from build123d import *

# Parameters (mm, degrees)
BOSS_EXTRU_1_DEPTH   = 6
EMPREINTE1_OUTLINE_W = 6
EMPREINTE1_OUTLINE_H = 18
EMPREINTE1_DEPTH     = 6


# Read off the part's stored shape, not the designer's step: Empreinte1
with BuildPart() as part:
    # Esquisse1 → Boss.-Extru.1 (new body)
    with BuildSketch(Plane.XY):
        Polygon((-286.806510123, 2.22734392), (-90.921937441, 115.321354688), (51.5, 33.094010768), (51.5, -193.094010768), (-90.921937441, -275.321354688), (-286.806510123, -162.22734392), align=None)
        Polygon((-246.806510123, -139.133333153), (-246.806510123, -20.866666847), (-90.921937441, 69.133333153), (11.5, 10), (11.5, -170), (-90.921937441, -229.133333153), align=None, mode=Mode.SUBTRACT)
    extrude(amount=BOSS_EXTRU_1_DEPTH)

    # Empreinte1 outline → Empreinte1 (cut)
    with BuildSketch(Plane.XY):
        Polygon((-6.833974392, -200.800909817), (-3.833974392, -205.99706224), (11.754482876, -196.99706224), (8.754482876, -191.800909817), align=None)
        Polygon((-22.42243166, -209.800909817), (-38.010888928, -218.800909817), (-35.010888928, -223.99706224), (-19.42243166, -214.99706224), align=None)
        Polygon((-53.599346196, -227.800909817), (-69.187803464, -236.800909817), (-66.187803464, -241.99706224), (-50.599346196, -232.99706224), align=None)
        with Locations((-266.319584862, -116.867002045)):
            Rectangle(EMPREINTE1_OUTLINE_W, EMPREINTE1_OUTLINE_H)
        with Locations((-266.319584862, -80.867002045)):
            Rectangle(EMPREINTE1_OUTLINE_W, EMPREINTE1_OUTLINE_H)
        with Locations((-266.319584862, -44.867002045)):
            Rectangle(EMPREINTE1_OUTLINE_W, EMPREINTE1_OUTLINE_H)
        Polygon((-54.593654623, 67.789098441), (-51.593654623, 72.985250863), (-67.182111891, 81.985250863), (-70.182111891, 76.789098441), align=None)
        Polygon((-39.005197355, 58.789098441), (-23.416740087, 49.789098441), (-20.416740087, 54.985250863), (-36.005197355, 63.985250863), align=None)
        Polygon((-7.828282819, 40.789098441), (7.76017445, 31.789098441), (10.76017445, 36.985250863), (-4.828282819, 45.985250863), align=None)
    extrude(amount=EMPREINTE1_DEPTH, mode=Mode.SUBTRACT)


solid = part.part
Verification items for the finished model (mm, model axes). A direction names the side the tool comes from. Coordinates: 2 decimals unless noted, no trailing zeros. Order: outer loops, then holes, each group sorted by start corner. A loop starts at its lowest first (then second) coordinate and runs counter-clockwise, first axis right, second up.
Item 1: Section check D-D, the plane z = 5. Give the number of separate pieces and of enclosed holes in the cut face, then the cut area to 3 significant figures.
Filled in:
separate pieces: 1
enclosed holes: 10
area: 40,400 mm2
Item 2: Release check for a two-part mould opening along X. For faces 1 (the face through (-154, -195, 6)), 2 (the face through (-190.24, 57.98, 2.96)), 3 (the face through (-59.279, 77.422, 2.958)) record: +X half, -X half, draft (parallel to the pull), parting line (faces both ways), or undercut.
Filled in:
face 1: draft
face 2: -X half
face 3: undercut
Item 3: Section check B-B, the plane x = -212.5. Enter the section's corners in (y, z).
Filled in:
outline: (-205.13, 0) - (-158.94, 0) - (-158.94, 6) - (-205.13, 6) - close; (-1.06, 0) - (45.13, 0) - (45.13, 6) - (-1.06, 6) - close
Item 4: Section check C-C, the plane y = -4. Enter the section's corners in (x, z), then the cut area to 3 significant figures.
Filled in:
outline: (-286.81, 0) - (-217.59, 0) - (-217.59, 6) - (-286.81, 6) - close; (11.5, 0) - (51.5, 0) - (51.5, 6) - (11.5, 6) - close
area: 655 mm2
Item 5: Access from +Z, -Z, +X, -X, +Y, -Y to the whole of each face (thin tool, end or side, straight path). Record for faces 4 (the face through (-18.71, -233.63, 2.96)), 5 (the face through (-0.14, 36.35, 2.96)).
Filled in:
face 4: +Z, -Z, +X, -Y
face 5: +Z, -Z
Item 6: Section check A-A, the plane y = -43.5. Enter the section's corners in (x, z).
Filled in:
outline: (-286.81, 0) - (-269.32, 0) - (-269.32, 6) - (-286.81, 6) - close; (-263.32, 0) - (-246.81, 0) - (-246.81, 6) - (-263.32, 6) - close; (11.5, 0) - (51.5, 0) - (51.5, 6) - (11.5, 6) - close
Item 7: Depth check by flat-ended pin: pin 1 (1.8 mm diameter, centred on x = -265.5, z = 3, fed in from -Y); pin 2 (3 mm diameter, centred on x = -266.5, z = 2.5, fed in from -Y); pin 3 (3 mm diameter, centred on x = -266, z = 4, fed in from +Y). Enter the tip coordinate at first touch or a pass-through.
Filled in:
pin 1: stops at y = -175.05
pin 2: stops at y = -174.82
pin 3: stops at y = 15.11
Item 8: Material ranges on L1, parallel to X at y = -109, z = 4.1; L2, parallel to Y at x = -58, z = 0.3; L3, parallel to X at y = -58, z = 0.9, recorded low to high.
Filled in:
L1: x = -286.81 to -269.32, -263.32 to -246.81, 11.5 to 51.5
L2: y = -256.31 to -237.27, -230.34 to -210.13, 50.13 to 69.76, 76.68 to 96.31
L3: x = -286.81 to -246.81, 11.5 to 51.5
